from build123d import *

# Parameters (mm, degrees)
F0_R     = 1
F3_DEPTH = 1
F4_DEPTH = 12
F2_R     = 7.92
F2_R_2   = 7.12
F5_DEPTH = 0.2
F6_DEPTH = 2


with BuildPart() as f3:
    # F0 (on Top) → F3 (new body)
    with BuildSketch(Plane.XY):
        with BuildLine():
            Line((-1, 7.7860452092), (-1, 7.1807033082))
            ThreePointArc((-1, 7.1807033082), (-5.1265241636, 5.1265241636), (-7.1807033082, 1))
            Line((-7.1807033082, 1), (-7.7860452092, 1))
            ThreePointArc((-7.7860452092, 1), (-7.85, 0), (-7.7860452092, -1))
            Line((-7.7860452092, -1), (-7.1807033082, -1))
            ThreePointArc((-7.1807033082, -1), (-5.1265241636, -5.1265241636), (-1, -7.1807033082))
            Line((-1, -7.1807033082), (-1, -7.7860452092))
            ThreePointArc((-1, -7.7860452092), (0, -7.85), (1, -7.7860452092))
            Line((1, -7.7860452092), (1, -7.1807033082))
            ThreePointArc((1, -7.1807033082), (5.1265241636, -5.1265241636), (7.1807033082, -1))
            Line((7.1807033082, -1), (7.7860452092, -1))
            ThreePointArc((7.7860452092, -1), (7.8339949864, -0.5010215103), (7.85, 0))
            ThreePointArc((7.85, 0), (7.8339949864, 0.5010215103), (7.7860452092, 1))
            Line((7.7860452092, 1), (7.1807033082, 1))
            ThreePointArc((7.1807033082, 1), (5.1265241636, 5.1265241636), (1, 7.1807033082))
            Line((1, 7.1807033082), (1, 7.7860452092))
            ThreePointArc((1, 7.7860452092), (0, 7.85), (-1, 7.7860452092))
        make_face()
        with BuildLine():
            Line((-6.1694813396, -1), (-5.153882032, -1))
            ThreePointArc((-5.153882032, -1), (-3.7123106012, -3.7123106012), (-1, -5.153882032))
            Line((-1, -5.153882032), (-1, -6.1694813396))
            ThreePointArc((-1, -6.1694813396), (-4.4194173824, -4.4194173824), (-6.1694813396, -1))
        make_face(mode=Mode.SUBTRACT)
        with BuildLine():
            ThreePointArc((-1, -4.1306779105), (-3.00520382, -3.00520382), (-4.1306779105, -1))
            Line((-4.1306779105, -1), (-3.0923292192, -1))
            ThreePointArc((-3.0923292192, -1), (-2.2980970389, -2.2980970389), (-1, -3.0923292192))
            Line((-1, -3.0923292192), (-1, -4.1306779105))
        make_face(mode=Mode.SUBTRACT)
        with BuildLine():
            ThreePointArc((-1, -2.0155644371), (-1.5909902577, -1.5909902577), (-2.0155644371, -1))
            Line((-2.0155644371, -1), (-1, -1))
            Line((-1, -1), (-1, -2.0155644371))
        make_face(mode=Mode.SUBTRACT)
        with BuildLine():
            ThreePointArc((6.1694813396, -1), (4.4194173824, -4.4194173824), (1, -6.1694813396))
            Line((1, -6.1694813396), (1, -5.153882032))
            ThreePointArc((1, -5.153882032), (3.7123106012, -3.7123106012), (5.153882032, -1))
            Line((5.153882032, -1), (6.1694813396, -1))
        make_face(mode=Mode.SUBTRACT)
        with BuildLine():
            Line((3.0923292192, -1), (4.1306779105, -1))
            ThreePointArc((4.1306779105, -1), (3.00520382, -3.00520382), (1, -4.1306779105))
            Line((1, -4.1306779105), (1, -3.0923292192))
            ThreePointArc((1, -3.0923292192), (2.2980970389, -2.2980970389), (3.0923292192, -1))
        make_face(mode=Mode.SUBTRACT)
        with BuildLine():
            Line((1, -1), (2.0155644371, -1))
            ThreePointArc((2.0155644371, -1), (1.5909902577, -1.5909902577), (1, -2.0155644371))
            Line((1, -2.0155644371), (1, -1))
        make_face(mode=Mode.SUBTRACT)
        with BuildLine():
            ThreePointArc((-2.0155644371, 1), (-1.5909902577, 1.5909902577), (-1, 2.0155644371))
            Line((-1, 2.0155644371), (-1, 1))
            Line((-1, 1), (-2.0155644371, 1))
        make_face(mode=Mode.SUBTRACT)
        with BuildLine():
            ThreePointArc((-1, 3.0923292192), (-2.2980970389, 2.2980970389), (-3.0923292192, 1))
            Line((-3.0923292192, 1), (-4.1306779105, 1))
            ThreePointArc((-4.1306779105, 1), (-3.00520382, 3.00520382), (-1, 4.1306779105))
            Line((-1, 4.1306779105), (-1, 3.0923292192))
        make_face(mode=Mode.SUBTRACT)
        with BuildLine():
            ThreePointArc((-6.1694813396, 1), (-4.4194173824, 4.4194173824), (-1, 6.1694813396))
            Line((-1, 6.1694813396), (-1, 5.153882032))
            ThreePointArc((-1, 5.153882032), (-3.7123106012, 3.7123106012), (-5.153882032, 1))
            Line((-5.153882032, 1), (-6.1694813396, 1))
        make_face(mode=Mode.SUBTRACT)
        Circle(F0_R, mode=Mode.SUBTRACT)
        with BuildLine():
            ThreePointArc((1, 2.0155644371), (1.5909902577, 1.5909902577), (2.0155644371, 1))
            Line((2.0155644371, 1), (1, 1))
            Line((1, 1), (1, 2.0155644371))
        make_face(mode=Mode.SUBTRACT)
        with BuildLine():
            Line((4.1306779105, 1), (3.0923292192, 1))
            ThreePointArc((3.0923292192, 1), (2.2980970389, 2.2980970389), (1, 3.0923292192))
            Line((1, 3.0923292192), (1, 4.1306779105))
            ThreePointArc((1, 4.1306779105), (3.00520382, 3.00520382), (4.1306779105, 1))
        make_face(mode=Mode.SUBTRACT)
        with BuildLine():
            Line((1, 5.153882032), (1, 6.1694813396))
            ThreePointArc((1, 6.1694813396), (4.4194173824, 4.4194173824), (6.1694813396, 1))
            Line((6.1694813396, 1), (5.153882032, 1))
            ThreePointArc((5.153882032, 1), (3.7123106012, 3.7123106012), (1, 5.153882032))
        make_face(mode=Mode.SUBTRACT)
    extrude(amount=-F3_DEPTH)

    # F0 (on Top) → F4 (join)
    with BuildSketch(Plane.XY):
        with BuildLine():
            ThreePointArc((8.1891696771, -1), (8.234778377, -0.5009242278), (8.25, 0))
            ThreePointArc((8.25, 0), (8.234778377, 0.5009242278), (8.1891696771, 1))
            Line((8.1891696771, 1), (8.1891696771, -1))
        make_face()
        with BuildLine():
            Line((8.1891696771, -1), (8.1891696771, 1))
            ThreePointArc((8.1891696771, 1), (0, 8.25), (-8.1891696771, 1))
            Line((-8.1891696771, 1), (-8.1891696771, -1))
            ThreePointArc((-8.1891696771, -1), (-5.8336309448, -5.8336309448), (-1, -8.1891696771))
            Line((-1, -8.1891696771), (1, -8.1891696771))
            ThreePointArc((1, -8.1891696771), (5.8336309448, -5.8336309448), (8.1891696771, -1))
        make_face()
        with BuildLine():
            ThreePointArc((-7.7860452092, 1), (-5.5507882323, 5.5507882323), (-1, 7.7860452092))
            ThreePointArc((-1, 7.7860452092), (0, 7.85), (1, 7.7860452092))
            ThreePointArc((1, 7.7860452092), (5.5507882323, 5.5507882323), (7.7860452092, 1))
            ThreePointArc((7.7860452092, 1), (7.8339949864, 0.5010215103), (7.85, 0))
            ThreePointArc((7.85, 0), (7.8339949864, -0.5010215103), (7.7860452092, -1))
            ThreePointArc((7.7860452092, -1), (5.5507882323, -5.5507882323), (1, -7.7860452092))
            ThreePointArc((1, -7.7860452092), (0, -7.85), (-1, -7.7860452092))
            ThreePointArc((-1, -7.7860452092), (-5.5507882323, -5.5507882323), (-7.7860452092, -1))
            ThreePointArc((-7.7860452092, -1), (-7.85, 0), (-7.7860452092, 1))
        make_face(mode=Mode.SUBTRACT)
        with BuildLine():
            Line((-8.1891696771, -1), (-8.1891696771, 1))
            ThreePointArc((-8.1891696771, 1), (-8.25, 0), (-8.1891696771, -1))
        make_face()
        with BuildLine():
            ThreePointArc((-1, -8.1891696771), (0, -8.25), (1, -8.1891696771))
            Line((1, -8.1891696771), (-1, -8.1891696771))
        make_face()
    extrude(amount=-F4_DEPTH)

    # F2 (on offset) → F5 (join)
    with BuildSketch(Plane.XY.offset(-11)):
        Circle(F2_R)
        Circle(F2_R_2, mode=Mode.SUBTRACT)
        Circle(F2_R_2)
        with BuildLine():
            add(Edge.make_bspline(
                [(-4.4, -0.4), (-4.1333333333, -0.4), (-3.8666666667, -0.4), (-3.6, -0.4)],
                knots=[0, 0, 0, 0, 1, 1, 1, 1], degree=3))
            add(Edge.make_bspline(
                [(-4.4, -0.4), (-4.4, -0.1333333333), (-4.4, 0.1333333333), (-4.4, 0.4)],
                knots=[0, 0, 0, 0, 1, 1, 1, 1], degree=3))
            add(Edge.make_bspline(
                [(-4.4, 0.4), (-4.1333333333, 0.4), (-3.8666666667, 0.4), (-3.6, 0.4)],
                knots=[0, 0, 0, 0, 1, 1, 1, 1], degree=3))
            add(Edge.make_bspline(
                [(-3.6, -0.4), (-3.6, -0.1333333333), (-3.6, 0.1333333333), (-3.6, 0.4)],
                knots=[0, 0, 0, 0, 1, 1, 1, 1], degree=3))
        make_face(mode=Mode.SUBTRACT)
        with BuildLine():
            add(Edge.make_bspline(
                [(4.4, -0.4), (4.1333333333, -0.4), (3.8666666667, -0.4), (3.6, -0.4)],
                knots=[0, 0, 0, 0, 1, 1, 1, 1], degree=3))
            add(Edge.make_bspline(
                [(3.6, -0.4), (3.6, -0.1333333333), (3.6, 0.1333333333), (3.6, 0.4)],
                knots=[0, 0, 0, 0, 1, 1, 1, 1], degree=3))
            add(Edge.make_bspline(
                [(4.4, 0.4), (4.1333333333, 0.4), (3.8666666667, 0.4), (3.6, 0.4)],
                knots=[0, 0, 0, 0, 1, 1, 1, 1], degree=3))
            add(Edge.make_bspline(
                [(4.4, -0.4), (4.4, -0.1333333333), (4.4, 0.1333333333), (4.4, 0.4)],
                knots=[0, 0, 0, 0, 1, 1, 1, 1], degree=3))
        make_face(mode=Mode.SUBTRACT)
    extrude(amount=-F5_DEPTH)

    # F2 (on offset) → F6 (join)
    with BuildSketch(Plane.XY.offset(-11)):
        with BuildLine():
            add(Edge.make_bspline(
                [(-4.4, -0.4), (-4.4, -0.1333333333), (-4.4, 0.1333333333), (-4.4, 0.4)],
                knots=[0, 0, 0, 0, 1, 1, 1, 1], degree=3))
            add(Edge.make_bspline(
                [(-4.4, -0.4), (-4.1333333333, -0.4), (-3.8666666667, -0.4), (-3.6, -0.4)],
                knots=[0, 0, 0, 0, 1, 1, 1, 1], degree=3))
            add(Edge.make_bspline(
                [(-3.6, -0.4), (-3.6, -0.1333333333), (-3.6, 0.1333333333), (-3.6, 0.4)],
                knots=[0, 0, 0, 0, 1, 1, 1, 1], degree=3))
            add(Edge.make_bspline(
                [(-4.4, 0.4), (-4.1333333333, 0.4), (-3.8666666667, 0.4), (-3.6, 0.4)],
                knots=[0, 0, 0, 0, 1, 1, 1, 1], degree=3))
        make_face()
        with BuildLine():
            add(Edge.make_bspline(
                [(3.6, -0.4), (3.6, -0.1333333333), (3.6, 0.1333333333), (3.6, 0.4)],
                knots=[0, 0, 0, 0, 1, 1, 1, 1], degree=3))
            add(Edge.make_bspline(
                [(4.4, -0.4), (4.1333333333, -0.4), (3.8666666667, -0.4), (3.6, -0.4)],
                knots=[0, 0, 0, 0, 1, 1, 1, 1], degree=3))
            add(Edge.make_bspline(
                [(4.4, -0.4), (4.4, -0.1333333333), (4.4, 0.1333333333), (4.4, 0.4)],
                knots=[0, 0, 0, 0, 1, 1, 1, 1], degree=3))
            add(Edge.make_bspline(
                [(4.4, 0.4), (4.1333333333, 0.4), (3.8666666667, 0.4), (3.6, 0.4)],
                knots=[0, 0, 0, 0, 1, 1, 1, 1], degree=3))
        make_face()
    extrude(amount=-F6_DEPTH)


solid = f3.part
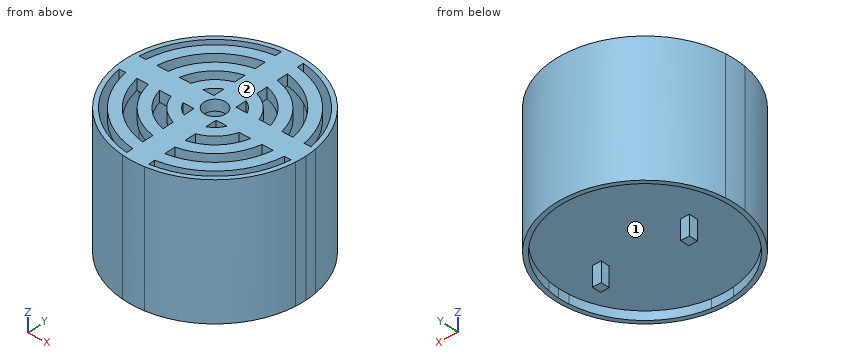
Verification items for the finished model (mm, model axes). Face numbers are marked on the shaded views. Coordinates: 2 decimals unless noted, no trailing zeros. Order: outer loops, then holes, each group sorted by start corner. A loop starts at its lowest first (then second) coordinate and runs counter-clockwise, first axis right, second up. Notation, with made-up numbers: (-23.5, -13.5) -> (12.5, -13.5) arc R17 cw to (12.5, 11.5) -> close; hole circle Ø7 at (70, 63.5). An arc over 180 degrees is marked (long way). Put each result on its own line as item: value. Start each with the question number.
1. Material ranges on L1, parallel to X at y = -1, z = -5.75; L2, parallel to Z at x = 4.5, y = 5.5; L3, parallel to Y at x = 0, z = -0.6, recorded low to high. Write a range as [from, to].
2. Cross-section at A-A, the plane z = -7.75. Record the boundary of the cut face in (x, y), then the cut area to 3 significant figures.
3. Cross-section at D-D, the plane y = -2.75. Count the separate pieces of the cut face and the enclosed holes in it, then the cut area to 3 significant figures.
4. Cross-section at C-C, the plane x = 0. Record the boundary of the cut face in (y, z).
5. Mould release check, pull along X, two halves, no side actions. Record for the marked faces 1 and 2: released by +X, released by -X, zero draft, split by the parting line, or undercut.
6. Go/stop test with flat-tipped pins: pin 1 Ø3 at (x, z) = (-6, -6.5) entering from -Y; pin 2 Ø1.1 at (x, z) = (3.5, -0.5) entering from +Y; pin 3 Ø1.5 at (y, z) = (3, -2.5) entering from -X. Record where each tip stops, or that it passes through.
7. Cross-section at B-B, the plane y = -4.75. Record the boundary of the cut face in (x, z), then the cut area to 3 significant figures.
Computed:
1. L1: [-8.19, -7.79], [7.79, 8.19]
1. L2: [-11.2, -11], [-1, 0]
1. L3: [-8.25, -1], [1, 8.25]
2. outline: circle Ø16.5 at (0, 0); hole circle Ø15.7 at (0, 0)
2. area: 20.2 mm2
3. separate pieces: 6
3. enclosed holes: 0
3. area: 21.3 mm2
4. outline: (-8.25, -12) -> (-7.85, -12) -> (-7.85, -11.2) -> (7.85, -11.2) -> (7.85, -12) -> (8.25, -12) -> (8.25, 0) -> (1, 0) -> (1, -1) -> (7.85, -1) -> (7.85, -11) -> (-7.85, -11) -> (-7.85, -1) -> (-1, -1) -> (-1, 0) -> (-8.25, 0) -> close
5. face 1: undercut
5. face 2: zero draft
6. pin 1: y = -6.91
6. pin 2: y = 7.7
6. pin 3: x = -7.94
7. outline: (-6.75, -12) -> (-6.25, -12) -> (-6.25, -11.2) -> (6.25, -11.2) -> (6.25, -12) -> (6.75, -12) -> (6.75, 0) -> (6.25, 0) -> (6.25, -11) -> (-6.25, -11) -> (-6.25, 0) -> (-6.75, 0) -> close; (-5.48, -1) -> (-4.06, -1) -> (-4.06, 0) -> (-5.48, 0) -> close; (-2.24, -1) -> (2.24, -1) -> (2.24, 0) -> (-2.24, 0) -> close; (4.06, -1) -> (5.48, -1) -> (5.48, 0) -> (4.06, 0) -> close
7. area: 21.7 mm2
